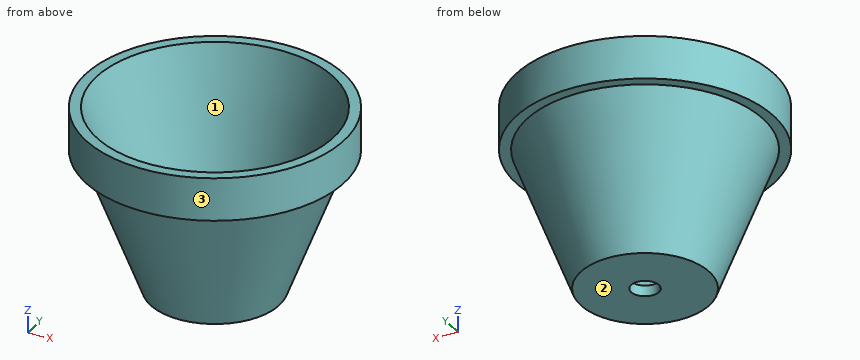
```python
from build123d import *

# Parameters (mm, degrees)
F2_R     = 3.25
F3_DEPTH = 42.676315


with BuildPart() as f1:
    # F0 (on Front) → F1 (revolve)
    with BuildSketch(Plane.XZ):
        Polygon((0, 2.5), (0, 0), (1.629259, 0), (15, 0), (27.542878, 32.675315), (30.042878, 32.675315), (30.042878, 42.675315), (27.542878, 42.675315), (13.875246, 2.5), (1.629259, 2.5), align=None)
    revolve(axis=Axis((0, 0, 21.337657), (0, 0, 1)))

    # F2 (on Top) → F3 (cut, through all)
    with BuildSketch(Plane.XY):
        Circle(F2_R)
    extrude(amount=F3_DEPTH, mode=Mode.SUBTRACT)


solid = f1.part
```
Can you work these out from the model? Positions are in its coordinate system, mm. Face numbers are marked on the shaded views. Coordinates: 2 decimals unless noted, no trailing zeros. Write each loop counter-clockwise with the first axis right and the second up, starting at its lowest first coordinate (ties: lowest second). Pieces come first, ordered by that corner, then holes. Notation, with made-up numbers: M 83,-19 L 88,-19 A21 ccw 88,19 Z; hole C 6,73.25 d1. An arc over 180 degrees is marked long. Write item = value, one per line. Start each with the question number.
Q1. If we section it at C-C, the plane z = 27.5: Write out the boundary of the cut face in (x, y).
Q2. Thinking about a two-plate mould opening in Y: for the marked faces 1, 2 and 3, which applies, released by +Y, released by -Y, zero draft, split by the parting line, or undercut?
Q3. I'm going to push flat-ended pins straight in: pin 1 (8.5 mm diameter, centred on x = 3, y = 2, fed in from +Z); pin 2 (5 mm diameter, centred on x = -8, z = 33, fed in from +Y); pin 3 (12 mm diameter, centred on y = -2, z = 34, fed in from -X); pin 4 (12 mm diameter, centred on y = 14, z = 10.5, fed in from +X). Where does each tip first touch, or does it pass through?
Q4. If we section it at A-A, the plane y = 0: Write out the boundary of the cut face in (x, z).
Q5. If I drill on L1, parallel to Z at x = -22, y = -17; L2, parallel to X at y = -7, z = 33; L3, parallel to Z at x = -12, y = -5, over which ranges is the centre line in solid material (lowest first)? Write a range as [from, to].
Check sheet entries:
q1.outline = C 0,0 d51.11; hole C 0,0 d44.76
q2.face_1 = undercut
q2.face_2 = zero draft
q2.face_3 = split by the parting line
q3.pin_1 = 2.5
q3.pin_2 = 29.54
q3.pin_3 = -30.04
q3.pin_4 = 18.23
q4.outline = M -30.04,32.68 L -27.54,32.68 L -15,0 L -3.25,0 L -3.25,2.5 L -13.88,2.5 L -27.54,42.68 L -30.04,42.68 Z; M 3.25,0 L 15,0 L 27.54,32.68 L 30.04,32.68 L 30.04,42.68 L 27.54,42.68 L 13.88,2.5 L 3.25,2.5 Z
q5.L1 = [32.68, 42.68]
q5.L2 = [-29.22, -23.22], [23.22, 29.22]
q5.L3 = [0, 2.5]
